Can you work these out from the model? Positions are in its coordinate system, mm. Face numbers are marked on the shaded views. A direction names the side the tool comes from. Give positions to 0.01 mm unless a question says otherwise; leave off trailing zeros. Order: outer loops, then holes, each group sorted by start corner. A loop starts at its lowest first (then second) coordinate and runs counter-clockwise, first axis right, second up. Notation, with made-up numbers: (36, -15) - (76, -15) arc R23 ccw to (76, 6) - close; hole circle Ø1 at (84.25, 21.5). An arc over 180 degrees is marked (long way). Answer as CSV lines item,"result".
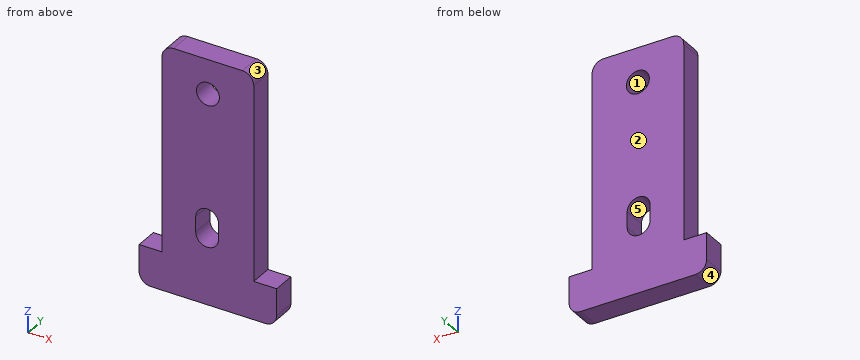
```python
from build123d import *

# Parameters (mm, degrees)
ESQUISSE1_W             = 18
ESQUISSE1_H             = 32
BOSS_EXTRU_1_DEPTH      = 3
ENL_V_MAT_EXTRU_1_REACH = 38.837
ESQUISSE2_W             = 3
ESQUISSE2_H             = 27
ENL_V_MAT_EXTRU_2_REACH = 38.837
ESQUISSE3_W             = 3
ESQUISSE3_H             = 27
ENL_V_MAT_EXTRU_3_REACH = 38.837
ESQUISSE4_R             = 1.5
CONG_1_R                = 1.5
CONG_2_R                = 1.5
ENL_V_MAT_EXTRU_4_REACH = 38.837


with BuildPart() as part:
    # Esquisse1 → Boss.-Extru.1 (new body)
    with BuildSketch(Plane(origin=(0, 0, 0), x_dir=(1, 0, 0), z_dir=(0, 1, 0))):
        with Locations((9, 16)):
            Rectangle(ESQUISSE1_W, ESQUISSE1_H)
    extrude(amount=BOSS_EXTRU_1_DEPTH)

    # Esquisse2 → Enlèv. mat.-Extru.1 (cut, up to next)
    with BuildSketch(Plane(origin=(0, 3, 0), x_dir=(1, 0, 0), z_dir=(0, 1, 0)), mode=Mode.PRIVATE) as enl_v_mat_extru_1_sk1:
        with Locations((1.5, 13.5)):
            Rectangle(ESQUISSE2_W, ESQUISSE2_H)
    enl_v_mat_extru_1_tool1 = extrude(enl_v_mat_extru_1_sk1.sketch, amount=-ENL_V_MAT_EXTRU_1_REACH, mode=Mode.PRIVATE) & part.part
    add(enl_v_mat_extru_1_tool1.solids().sort_by_distance((1.5, 3, -13.5))[0], mode=Mode.SUBTRACT)

    # Esquisse3 → Enlèv. mat.-Extru.2 (cut, up to next)
    with BuildSketch(Plane(origin=(0, 3, 0), x_dir=(1, 0, 0), z_dir=(0, 1, 0)), mode=Mode.PRIVATE) as enl_v_mat_extru_2_sk1:
        with Locations((16.5, 13.5)):
            Rectangle(ESQUISSE3_W, ESQUISSE3_H)
    enl_v_mat_extru_2_tool1 = extrude(enl_v_mat_extru_2_sk1.sketch, amount=-ENL_V_MAT_EXTRU_2_REACH, mode=Mode.PRIVATE) & part.part
    add(enl_v_mat_extru_2_tool1.solids().sort_by_distance((16.5, 3, -13.5))[0], mode=Mode.SUBTRACT)

    # Esquisse4 → Enlèv. mat.-Extru.3 (cut, up to next)
    with BuildSketch(Plane(origin=(0, 3, 0), x_dir=(1, 0, 0), z_dir=(0, 1, 0)), mode=Mode.PRIVATE) as enl_v_mat_extru_3_sk1:
        with Locations(Location((9, 4.5, 0), (0, 0, 270))):
            Circle(ESQUISSE4_R)
    enl_v_mat_extru_3_tool1 = extrude(enl_v_mat_extru_3_sk1.sketch, amount=-ENL_V_MAT_EXTRU_3_REACH, mode=Mode.PRIVATE) & part.part
    add(enl_v_mat_extru_3_tool1.solids().sort_by_distance((9, 3, -4.5))[0], mode=Mode.SUBTRACT)

    # Congé1
    cong_1_edges = [part.edges().sort_by_distance(p)[0] for p in [
        (0, 1.5, -32),
        (18, 1.5, -32),
    ]]
    fillet(cong_1_edges, radius=CONG_1_R)

    # Congé2
    cong_2_edges = [part.edges().sort_by_distance(p)[0] for p in [
        (3, 1.5, 0),
        (15, 1.5, 0),
    ]]
    fillet(cong_2_edges, radius=CONG_2_R)

    # Esquisse5 → Enlèv. mat.-Extru.4 (cut, up to next)
    with BuildSketch(Plane(origin=(0, 3, 0), x_dir=(1, 0, 0), z_dir=(0, 1, 0)), mode=Mode.PRIVATE) as enl_v_mat_extru_4_sk1:
        with BuildLine():
            Line((10.403583012, 23), (10.403583012, 21))
            ThreePointArc((10.403583012, 21), (8.903583012, 19.5), (7.403583012, 21))
            Line((7.403583012, 21), (7.403583012, 23))
            ThreePointArc((7.403583012, 23), (8.903583012, 24.5), (10.403583012, 23))
        make_face()
    enl_v_mat_extru_4_tool1 = extrude(enl_v_mat_extru_4_sk1.sketch, amount=-ENL_V_MAT_EXTRU_4_REACH, mode=Mode.PRIVATE) & part.part
    add(enl_v_mat_extru_4_tool1.solids().sort_by_distance((8.903583, 3, -22))[0], mode=Mode.SUBTRACT)


solid = part.part
```
1) I want a section at C-C on y = 2.55. Write out the boundary of the cut face in (x, z).
Answer block:
outline,"(0, -30.5) arc R1.5 ccw to (1.5, -32) - (16.5, -32) arc R1.5 ccw to (18, -30.5) - (18, -27) - (15, -27) - (15, -1.5) arc R1.5 ccw to (13.5, 0) - (4.5, 0) arc R1.5 ccw to (3, -1.5) - (3, -27) - (0, -27) - close; hole (7.4, -23) arc R1.5 ccw to (10.4, -23) - (10.4, -21) arc R1.5 ccw to (7.4, -21) - close; hole circle Ø3 at (9, -4.5)"
2) If we mould it in two halves opening along X, with no side actions, what happens to the marked faces 1, 2 and 3? For each: +X half, -X half, draft (parallel to the pull), parting line (faces both ways), or undercut.
Answer block:
face 1,"undercut"
face 2,"draft"
face 3,"+X half"
3) I want a section at A-A on z = -4.5. Write out the boundary of the cut face in (x, y).
Answer block:
outline,"(3, 0) - (7.5, 0) - (7.5, 3) - (3, 3) - close; (10.5, 0) - (15, 0) - (15, 3) - (10.5, 3) - close"
4) I need wall thicknesses on line 1 along X through (y, z) = (2, -4.5); line 2 along X through (y, z) = (1.5, -13); line 3 along Z through (x, y) = (2.5, 0.9). Which ranges of each line are inside material? Lowest first, please. Write a range as [from, to].
Answer block:
line 1,"[3, 7.5], [10.5, 15]"
line 2,"[3, 15]"
line 3,"[-32, -27]"
5) I want a section at B-B on x = 8.5. Write out the boundary of the cut face in (y, z).
Answer block:
outline,"(0, -32) - (3, -32) - (3, -24.44) - (0, -24.44) - close; (0, -19.56) - (3, -19.56) - (3, -5.91) - (0, -5.91) - close; (0, -3.09) - (3, -3.09) - (3, 0) - (0, 0) - close"
6) I want a section at D-D on z = -17. Write out the boundary of the cut face in (x, y), plus the area to 3 significant figures.
Answer block:
outline,"(3, 0) - (15, 0) - (15, 3) - (3, 3) - close"
area,"36.0 mm2"
7) I'm going to push flat-ended pins straight in: P1, Ø1, axis at y = 2, z = -13, coming from the +X side; P2, Ø1.5, axis at y = 1, z = -10.5, coming from the -X side; P3, Ø0.9, axis at x = 16.5, y = 1, coming from the +Z side. Where does each tip first touch, or does it pass through?
Answer block:
P1,"x = 15"
P2,"x = 3"
P3,"z = -27"
8) Which directions (+Z, -Z, +X, -X, +Y, -Y) give clear straight access to the entire face, cutting with the end or side of a thin tool? Please do the marked faces 4 and 5.
Answer block:
face 4,"-Z, -X, +Y, -Y"
face 5,"+Y, -Y"
